Design review of the part built by this model. Coordinates are the model's own, in mm. Round coordinates to 2 decimals unless told otherwise and drop trailing zeros. Order: outer loops, then holes, each group sorted by start corner. A loop starts at its lowest first (then second) coordinate and runs counter-clockwise, first axis right, second up. Notation, with made-up numbers: M 44.25,80 L 93.25,80 A11 ccw 93.25,93 Z; hole C 6.5,19.25 d8. An arc over 180 degrees is marked long. Use a Markdown table: item, result. Add a question column.
(1) The part is to be moulded in two halves that separate along X. For faces 1 (the face through (7.5, -3, 0)), 2 (the face through (-0.65, -3.13, 33.32)), 3 (the face through (0, -6.35, 0)), say which applies: released by +X, released by -X, zero draft, split by the parting line, or undercut.
(2) Take a section at C-C (y = -3.75). Write out the cut boundary in (x, z) (3 decimals), then the cut area to 3 significant figures.
(3) Take a section at A-A (x = 0). Write out the cut boundary in (y, z) (3 decimals).
(4) To check wall thickness, follow probe 1 along X at (y, z) = (-2.25, 25); probe 2 along Z at (x, y) = (0, -4.75) (3 decimals); probe 3 along X at (y, z) = (-2.5, 28). State the ranges of each line that lie inside material, in increasing order. Write a range as from..to.
(5) Take a section at B-B (z = 27.5). Write out the cut boundary in (x, y).
(6) For pin 1 (1 mm diameter, centred on x = -2, z = 9, fed in from +Y); pin 2 (1 mm diameter, centred on x = -3.5, z = 26, fed in from +Y), all flat-tipped, find the tip position at first contact; note any pin that passes through.
```python
from build123d import *

# Parameters (mm, degrees)
F0_R     = 5
F1_DEPTH = 6.35


with BuildPart() as f1:
    # F0 (on Front) → F1 (new body)
    with BuildSketch(Plane.XZ):
        with BuildLine():
            Line((3.69, 34.925), (-3.69, 34.925))
            ThreePointArc((-3.69, 34.925), (-6.384077, 33.809077), (-7.5, 31.115))
            Line((-7.5, 31.115), (-7.5, -31.115))
            ThreePointArc((-7.5, -31.115), (-6.384077, -33.809077), (-3.69, -34.925))
            Line((-3.69, -34.925), (3.69, -34.925))
            ThreePointArc((3.69, -34.925), (6.384077, -33.809077), (7.5, -31.115))
            Line((7.5, -31.115), (7.5, 31.115))
            ThreePointArc((7.5, 31.115), (6.384077, 33.809077), (3.69, 34.925))
        make_face()
        with Locations((0, 28.362114)):
            Circle(F0_R, mode=Mode.SUBTRACT)
    extrude(amount=F1_DEPTH)


solid = f1.part
```
Verdict:
| question | item | result |
|---|---|---|
| 1 | face 1 | released by +X |
| 1 | face 2 | undercut |
| 1 | face 3 | zero draft |
| 2 | outline | M -7.5,-31.115 A3.81 ccw -3.69,-34.925 L 3.69,-34.925 A3.81 ccw 7.5,-31.115 L 7.5,31.115 A3.81 ccw 3.69,34.925 L -3.69,34.925 A3.81 ccw -7.5,31.115 Z; hole C 0,28.362 d10 |
| 2 | area | 957 mm^2 |
| 3 | outline | M -6.35,-34.925 L 0,-34.925 L 0,23.362 L -6.35,23.362 Z; M -6.35,33.362 L 0,33.362 L 0,34.925 L -6.35,34.925 Z |
| 4 | probe 1 | x = -7.5..-3.7, 3.7..7.5 |
| 4 | probe 2 | z = -34.925..23.362, 33.362..34.925 |
| 4 | probe 3 | x = -7.5..-4.99, 4.99..7.5 |
| 5 | outline | M -7.5,-6.35 L -4.93,-6.35 L -4.93,0 L -7.5,0 Z; M 4.93,-6.35 L 7.5,-6.35 L 7.5,0 L 4.93,0 Z |
| 6 | pin 1 | stops at y = 0 |
| 6 | pin 2 | passes through |
